Geometry check sheet. Reference: the model listing, model coordinates, mm. A direction names the side the tool comes from. Round coordinates to 2 decimals unless told otherwise and drop trailing zeros. Write each loop counter-clockwise with the first axis right and the second up, starting at its lowest first coordinate (ties: lowest second). Pieces come first, ordered by that corner, then holes. Notation, with made-up numbers: (28.25, 18.5) - (45.25, 18.5) arc R32 ccw to (45.25, 57.5) - close; hole circle Ø9 at (75, 89). An arc over 180 degrees is marked (long way). One line per question, with ' | ' between items. Start each with the question number.
from build123d import *

# Parameters (mm, degrees)
SZKIC1_R                    = 2.5
DODANIE_WYCI_GNI_CIE1_DEPTH = 6.3


with BuildPart() as part:
    # Szkic1 → Dodanie-wyciągnięcie1 (new body)
    with BuildSketch(Plane.XY):
        with BuildLine():
            Line((0.875, 5.423398291), (0.775, 3.822221213))
            ThreePointArc((0.775, 3.822221213), (1.492465386, 3.603130177), (2.154710783, 3.250726294))
            Line((2.154710783, 3.250726294), (3.216203275, 4.453640142))
            Line((3.216203275, 4.453640142), (4.245186445, 4.844987722))
            ThreePointArc((4.245186445, 4.844987722), (4.453444634, 4.765560203), (4.631549417, 4.631549417))
            ThreePointArc((4.631549417, 4.631549417), (4.765560203, 4.453444634), (4.844987722, 4.245186445))
            Line((4.844987722, 4.245186445), (4.453640142, 3.216203275))
            Line((4.453640142, 3.216203275), (3.250726294, 2.154710783))
            ThreePointArc((3.250726294, 2.154710783), (3.603130177, 1.492465386), (3.822221213, 0.775))
            Line((3.822221213, 0.775), (5.423398291, 0.875))
            Line((5.423398291, 0.875), (6.427723795, 0.424123551))
            ThreePointArc((6.427723795, 0.424123551), (6.518820836, 0.220699035), (6.55, 0))
            ThreePointArc((6.55, 0), (6.518820836, -0.220699035), (6.427723795, -0.424123551))
            Line((6.427723795, -0.424123551), (5.423398291, -0.875))
            Line((5.423398291, -0.875), (3.822221213, -0.775))
            ThreePointArc((3.822221213, -0.775), (3.603130177, -1.492465386), (3.250726294, -2.154710783))
            Line((3.250726294, -2.154710783), (4.453640142, -3.216203275))
            Line((4.453640142, -3.216203275), (4.844987722, -4.245186445))
            ThreePointArc((4.844987722, -4.245186445), (4.765560203, -4.453444634), (4.631549417, -4.631549417))
            ThreePointArc((4.631549417, -4.631549417), (4.453444634, -4.765560203), (4.245186445, -4.844987722))
            Line((4.245186445, -4.844987722), (3.216203275, -4.453640142))
            Line((3.216203275, -4.453640142), (2.154710783, -3.250726294))
            ThreePointArc((2.154710783, -3.250726294), (1.492465386, -3.603130177), (0.775, -3.822221213))
            Line((0.775, -3.822221213), (0.875, -5.423398291))
            Line((0.875, -5.423398291), (0.424123551, -6.427723795))
            ThreePointArc((0.424123551, -6.427723795), (0.220699035, -6.518820836), (0, -6.55))
            ThreePointArc((0, -6.55), (-0.220699035, -6.518820836), (-0.424123551, -6.427723795))
            Line((-0.424123551, -6.427723795), (-0.875, -5.423398291))
            Line((-0.875, -5.423398291), (-0.775, -3.822221213))
            ThreePointArc((-0.775, -3.822221213), (-1.492465386, -3.603130177), (-2.154710783, -3.250726294))
            Line((-2.154710783, -3.250726294), (-3.216203275, -4.453640142))
            Line((-3.216203275, -4.453640142), (-4.245186445, -4.844987722))
            ThreePointArc((-4.245186445, -4.844987722), (-4.453444634, -4.765560203), (-4.631549417, -4.631549417))
            ThreePointArc((-4.631549417, -4.631549417), (-4.765560203, -4.453444634), (-4.844987722, -4.245186445))
            Line((-4.844987722, -4.245186445), (-4.453640142, -3.216203275))
            Line((-4.453640142, -3.216203275), (-3.250726294, -2.154710783))
            ThreePointArc((-3.250726294, -2.154710783), (-3.603130177, -1.492465386), (-3.822221213, -0.775))
            Line((-3.822221213, -0.775), (-5.423398291, -0.875))
            Line((-5.423398291, -0.875), (-6.427723795, -0.424123551))
            ThreePointArc((-6.427723795, -0.424123551), (-6.518820836, -0.220699035), (-6.55, 0))
            ThreePointArc((-6.55, 0), (-6.518820836, 0.220699035), (-6.427723795, 0.424123551))
            Line((-6.427723795, 0.424123551), (-5.423398291, 0.875))
            Line((-5.423398291, 0.875), (-3.822221213, 0.775))
            ThreePointArc((-3.822221213, 0.775), (-3.603130177, 1.492465386), (-3.250726294, 2.154710783))
            Line((-3.250726294, 2.154710783), (-4.453640142, 3.216203275))
            Line((-4.453640142, 3.216203275), (-4.844987722, 4.245186445))
            ThreePointArc((-4.844987722, 4.245186445), (-4.765560203, 4.453444634), (-4.631549417, 4.631549417))
            ThreePointArc((-4.631549417, 4.631549417), (-4.453444634, 4.765560203), (-4.245186445, 4.844987722))
            Line((-4.245186445, 4.844987722), (-3.216203275, 4.453640142))
            Line((-3.216203275, 4.453640142), (-2.154710783, 3.250726294))
            ThreePointArc((-2.154710783, 3.250726294), (-1.492465386, 3.603130177), (-0.775, 3.822221213))
            Line((-0.775, 3.822221213), (-0.875, 5.423398291))
            Line((-0.875, 5.423398291), (-0.424123551, 6.427723795))
            ThreePointArc((-0.424123551, 6.427723795), (-0.220699035, 6.518820836), (0, 6.55))
            ThreePointArc((0, 6.55), (0.220699035, 6.518820836), (0.424123551, 6.427723795))
            Line((0.424123551, 6.427723795), (0.875, 5.423398291))
        make_face()
        Circle(SZKIC1_R, mode=Mode.SUBTRACT)
    extrude(amount=DODANIE_WYCI_GNI_CIE1_DEPTH)


solid = part.part
Q1. Section check B-B, the plane y = 3. Record the cut outline in (x, z).
Q2. Set-up check for faces 1 (the flat face through (-4.647, 3.723, 3.106)), 2 (the flat face through (-4.634, 0.826, 3.106)), 3 (the flat face through (-3.723, -4.647, 3.106)): record each of +Z, -Z, +X, -X, +Y, -Y from which the full face is reachable in a straight line by a thin tool's end or side.
Q3. Go/stop test with flat-tipped pins: P1, Ø3, axis at x = 1, y = -5, coming from the +Z side; P2, Ø1, axis at y = -2.5, z = 4.5, coming from the +X side; P3, Ø1.5, axis at x = -2, z = 3.5, coming from the +Y side. Record where each tip stops, or that it passes through.
Q4. Draft check along Y on faces 4 (the flat face through (-5.92, -0.65, 3.11)), 5 (the flat face through (0.646, 5.933, 3.106)), 6 (the flat face through (4.612, 0.824, 3.106)). Enter one of: pulls with the +Y half, pulls with the -Y half, needs draft (parallel to the pull), parting line crosses it, or undercut.
Q5. Section check A-A, the plane y = -4. Record the cut outline in (x, z).
Q6. Thickness scan on line 1 (X direction, y = -1.25, z = 5.25); line 2 (Y direction, x = 1, z = 2.75); line 3 (X direction, y = 3.5, z = 4.25). Record the ranges inside material, lowest first.
Result sheet:
1) outline: (-4.21, 0) - (4.21, 0) - (4.21, 6.3) - (-4.21, 6.3) - close
2) face 1: +Z, -Z, -X | face 2: +Z, -Z | face 3: +Z, -Z, -Y
3) P1: z = 6.3 | P2: x = 4.21 | P3: y = 3.93
4) face 4: pulls with the -Y half | face 5: pulls with the +Y half | face 6: undercut
5) outline: (-4.75, 0) - (-2.82, 0) - (-2.82, 6.3) - (-4.75, 6.3) - close; (-0.79, 0) - (0.79, 0) - (0.79, 6.3) - (-0.79, 6.3) - close; (2.82, 0) - (4.75, 0) - (4.75, 6.3) - (2.82, 6.3) - close
6) line 1: -3.69 to -2.17, 2.17 to 3.69 | line 2: -3.77 to -2.29, 2.29 to 3.77 | line 3: -4.56 to -2.37, -1.72 to 1.72, 2.37 to 4.56
